```python
from build123d import *
from build123d.topology import SkipClean

# Parameters (mm, degrees)
SKETCH1_W           = 8
SKETCH1_H           = 5
BOSS_EXTRUDE1_DEPTH = 2.5
SKETCH2_W           = 3
SKETCH2_H           = 3
BOSS_EXTRUDE2_DEPTH = 1.5
CUT_EXTRUDE2_DEPTH  = 3
SKETCH5_R           = 1.2
CUT_EXTRUDE3_DEPTH  = 9.440971508
BOSS_EXTRUDE3_START = 15
SKETCH6_R           = 1.5
BOSS_EXTRUDE3_DEPTH = 15


with BuildPart() as part:
    # Sketch1 → Boss-Extrude1 (new, symmetric)
    with BuildSketch(Plane(origin=(0, 0, 0), x_dir=(1, 0, 0), z_dir=(0, 1, 0))):
        Rectangle(SKETCH1_W, SKETCH1_H)
    extrude(amount=BOSS_EXTRUDE1_DEPTH, both=True)

    # Sketch2 → Boss-Extrude2 (add, symmetric)
    with BuildSketch(Plane(origin=(0, 0, 0), x_dir=(1, 0, 0), z_dir=(0, 1, 0))):
        with Locations((0, -4)):
            Rectangle(SKETCH2_W, SKETCH2_H)
    extrude(amount=BOSS_EXTRUDE2_DEPTH, both=True)

    # Sketch3 → Cut-Extrude2 (cut)
    with BuildSketch(Plane.XY.offset(5.5)):
        with BuildLine():
            Line((-1.5, 1.5), (-1.5, 0))
            ThreePointArc((-1.5, 0), (-1.060660172, 1.060660172), (0, 1.5))
            Line((0, 1.5), (-1.5, 1.5))
        make_face()
        with BuildLine():
            ThreePointArc((0, 1.5), (1.060660172, 1.060660172), (1.5, 0))
            Line((1.5, 0), (1.5, 1.5))
            Line((1.5, 1.5), (0, 1.5))
        make_face()
        with BuildLine():
            ThreePointArc((1.5, 0), (1.060660172, -1.060660172), (0, -1.5))
            Line((0, -1.5), (1.5, -1.5))
            Line((1.5, -1.5), (1.5, 0))
        make_face()
        with BuildLine():
            Line((-1.5, 0), (-1.5, -1.5))
            Line((-1.5, -1.5), (0, -1.5))
            ThreePointArc((0, -1.5), (-1.060660172, -1.060660172), (-1.5, 0))
        make_face()
    extrude(amount=-CUT_EXTRUDE2_DEPTH, mode=Mode.SUBTRACT)

    # Sketch5 → Cut-Extrude3 (cut, through all)
    with BuildSketch(Plane(origin=(0, 2.5, 0), x_dir=(1, 0, 0), z_dir=(0, 1, 0))):
        with Locations(Location((0, 0, 0), (0, 0, 270))):
            Circle(SKETCH5_R)
    extrude(amount=-CUT_EXTRUDE3_DEPTH, mode=Mode.SUBTRACT)

    # Sketch6 → Boss-Extrude3 (add)
    with SkipClean():  # the faces are left unmerged after this step: merging them gives an invalid solid
        with BuildSketch(Plane.XY.offset(5.5).offset(BOSS_EXTRUDE3_START)):
            Circle(SKETCH6_R)
        extrude(amount=-BOSS_EXTRUDE3_DEPTH)


solid = part.part
```
The listing builds one solid part. Answer for the finished solid, in the listing's coordinates (mm). Coordinates: 2 decimals unless noted, no trailing zeros. Write each loop counter-clockwise with the first axis right and the second up, starting at its lowest first coordinate (ties: lowest second). Pieces come first, ordered by that corner, then holes. Notation, with made-up numbers: (-3, -28) - (30, -28) arc R23 cw to (30, -18) - close; hole circle Ø9 at (37.5, 55.5). An arc over 180 degrees is marked (long way). Return JSON: item names as keys, results as strings. Group by question number.
Q1. For a pull along X with two mould halves and no side action, classify faces 1 (the cylindrical face through (1.01, 0.04, 0.65)), 2 (the flat face through (0, 2, 2.5)), 3 (the flat face through (4, 0, 0)) as +X half, -X half, draft (parallel to the pull), parting line (faces both ways), or undercut.
Q2. The part is cut by section C-C on x = -1. Write down the section's boundary in (y, z).
Q3. The part is cut by section A-A on z = 0. Write down the section's boundary in (x, y), and give its area (3 significant figures).
Q4. The part is cut by section D-D on x = -2. Write down the section's boundary in (y, z).
Q5. Flat-ended cylindrical pins translate along their axes: pin 1 Ø1.5 at (x, y) = (-2, 2) entering from +Z; pin 2 Ø2 at (x, z) = (1, 13.5) entering from +Y; pin 3 Ø1.5 at (y, z) = (1, 8) entering from -X. Find the tip coordinate at first contact, or state that the pin passes through.
Q6. Find the intervals of material crossed by line 1 along X through (y, z) = (0.2, 0); line 2 along Y through (x, z) = (0, 15.5); line 3 along Z through (x, y) = (2.25, 0.9), in increasing order. Write a range as [from, to].
Q7. The part is cut by section B-B on y = -0.2. Write down the section's boundary in (x, z), and give its area (3 significant figures).
Evaluation:
{
 "1": {"face 1": "undercut", "face 2": "draft", "face 3": "+X half"},
 "2": {"outline": "(-2.5, -2.5) - (2.5, -2.5) - (2.5, -0.66) - (-2.5, -0.66) - close; (-2.5, 0.66) - (2.5, 0.66) - (2.5, 2.5) - (1.12, 2.5) - (1.12, 20.5) - (-1.12, 20.5) - (-1.12, 2.5) - (-2.5, 2.5) - close"},
 "3": {"outline": "(-4, -2.5) - (-1.2, -2.5) - (-1.2, 2.5) - (-4, 2.5) - close; (1.2, -2.5) - (4, -2.5) - (4, 2.5) - (1.2, 2.5) - close", "area": "28.0 mm2"},
 "4": {"outline": "(-2.5, -2.5) - (2.5, -2.5) - (2.5, 2.5) - (-2.5, 2.5) - close"},
 "5": {"pin 1": "stops at z = 2.5", "pin 2": "stops at y = 1.5", "pin 3": "stops at x = -1.48"},
 "6": {"line 1": "x = [-4, -1.2], [1.2, 4]", "line 2": "y = [-1.5, 1.5]", "line 3": "z = [-2.5, 2.5]"},
 "7": {"outline": "(-4, -2.5) - (4, -2.5) - (4, 2.5) - (1.49, 2.5) - (1.49, 20.5) - (-1.49, 20.5) - (-1.49, 2.5) - (-4, 2.5) - close; hole circle Ø2.4 at (0, 0)", "area": "89.0 mm2"}
}
